Work out the finished part from the listing and answer in its coordinate system (mm). A direction names the side the tool comes from. Round coordinates to 2 decimals unless told otherwise and drop trailing zeros. Write each loop counter-clockwise with the first axis right and the second up, starting at its lowest first coordinate (ties: lowest second). Pieces come first, ordered by that corner, then holes.
1. Find section B-B (x = -13.2). Write down the section's boundary in (y, z).
2. Find section A-A (y = -3). Write down the section's boundary in (x, z), and give its area (3 significant figures).
3. Find section C-C (z = -16). Write down the section's boundary in (x, y), and give its area (3 significant figures).
4. Determine the mould class of faces 1 (the face through (21.58, 3.46, -15.17)), 2 (the face through (-16, 1, -17)), 3 (the face through (-7.6, -7.43, -15.93)) for opening direction X: pulls with the +X half, pulls with the -X half, needs draft (parallel to the pull), parting line crosses it, or undercut.
5. Flat-ended cylindrical pins translate along their axes: pin 1 Ø6 at (x, z) = (-10.5, -16) entering from -Y; pin 2 Ø2.5 at (y, z) = (-3, -16.5) entering from +X; pin 3 Ø6 at (x, y) = (-10.5, -5.5) entering from +Z; pin 4 Ø5 at (y, z) = (-2.5, -16.5) entering from -X. Find the tip coordinate at first contact, or state that the pin passes through.
6. A tool of negligible diameter and unlimited length cuts with its end or side. For faces 4 (the face through (20, 6, -16)), 5 (the face through (-8.2, -3, -16)), 6 (the face through (19.2, -3, -16)), 7 (the face through (6, -6, -16)), from which of +Z, -Z, +X, -X, +Y, -Y can it reach the whole face along a straight path? Write none if from no direction.
7. Find section D-D (y = 3.5). Write down the section's boundary in (x, z).
8. Straight lines are drawn through the part: probe 1 along X at (y, z) = (4.35, -16); probe 2 along Z at (x, y) = (-13.2, 4.1); probe 3 along X at (y, z) = (2.4, -16). For each, find the intervals that lie inside material, in ascending order.
```python
from build123d import *

# Parameters (mm, degrees)
PAD053_DEPTH            = 5
SKETCH104_R             = 2.75
POCKET052_DEPTH         = 8.001
POCKET052_DEPTH_BACK    = 6.001
BODY032_PLACEMENT_ANGLE = 180


with BuildPart() as part:
    # Sketch103 → Pad053 (new body, symmetric)
    with BuildSketch(Plane(origin=(6, -6, 0), x_dir=(1, 0, 0), z_dir=(0, 0, 1))):
        with BuildLine():
            Line((-21.7, 5), (-15.7, 5))
            ThreePointArc((-15.7, 5), (-14.2857864376, 5.5857864376), (-13.7, 7))
            Line((-13.7, 7), (-13.7, 12))
            ThreePointArc((-11.7, 14), (-13.1142135624, 13.4142135624), (-13.7, 12))
            Line((-11.7, 14), (0, 14))
            Line((0, 14), (0, 12))
            Line((0, 12), (-11.7, 12))
            Line((-11.7, 12), (-11.7, 0))
            Line((-11.7, 0), (-23.7, 0))
            Line((-23.7, 0), (-23.7, 3))
            ThreePointArc((-21.7, 5), (-23.1142135624, 4.4142135624), (-23.7, 3))
        make_face()
    extrude(amount=PAD053_DEPTH, both=True)

    # Sketch104 → Pocket052 (cut, two sides)
    with BuildSketch(Plane.XZ) as pocket052_sk:
        with Locations((-12.7, 0)):
            Circle(SKETCH104_R)
    extrude(amount=-POCKET052_DEPTH, mode=Mode.SUBTRACT)
    extrude(pocket052_sk.sketch, amount=POCKET052_DEPTH_BACK, mode=Mode.SUBTRACT)

    # Mirrored024: part across Sketch103 V_Axis


with BuildPart() as part_1:
    add(part.part)
    add(part.part.mirror(Plane(origin=(6, -6, 0), x_dir=(0, 0, 1), z_dir=(1, 0, 0))))


with BuildPart() as part_2:
    # Body032 placement: moved
    add(part_1.part.moved(Location((11.5, 0, -16))).rotate(Axis((11.5, 0, -16), (0, 0, 1)), BODY032_PLACEMENT_ANGLE))


solid = part_2.part
```
Worked answers:
1. outline: (1, -21) - (6, -21) - (6, -18.75) - (1, -18.75) - close; (1, -13.25) - (6, -13.25) - (6, -11) - (1, -11) - close
2. outline: (-8.2, -21) - (-6.2, -21) - (-6.2, -11) - (-8.2, -11) - close; (17.2, -21) - (19.2, -21) - (19.2, -11) - (17.2, -11) - close
2. area: 40.0 mm2
3. outline: (-18.2, 3) arc R2 ccw to (-16.2, 1) - (-15.95, 1) - (-15.95, 6) - (-18.2, 6) - close; (-10.45, 1) - (-10.2, 1) arc R2 cw to (-8.2, -1) - (-8.2, -6) arc R2 ccw to (-6.2, -8) - (17.2, -8) arc R2 ccw to (19.2, -6) - (19.2, -1) arc R2 cw to (21.2, 1) - (21.45, 1) - (21.45, 6) - (17.2, 6) - (17.2, -6) - (-6.2, -6) - (-6.2, 6) - (-10.45, 6) - close; (26.95, 1) - (27.2, 1) arc R2 ccw to (29.2, 3) - (29.2, 6) - (26.95, 6) - close
3. area: 146 mm2
4. face 1: undercut
4. face 2: needs draft
4. face 3: pulls with the -X half
5. pin 1: stops at y = -7.52
5. pin 2: stops at x = 19.2
5. pin 3: stops at z = -11
5. pin 4: stops at x = -8.47
6. face 4: +Z, -Z, +X, -X, +Y
6. face 5: +Z, -Z, -X, -Y
6. face 6: +Z, -Z, +X, -Y
6. face 7: +Z, -Z, +Y
7. outline: (-18.2, -21) - (-6.2, -21) - (-6.2, -11) - (-18.2, -11) - close; (17.2, -21) - (29.2, -21) - (29.2, -11) - (17.2, -11) - close; hole circle Ø5.5 at (-13.2, -16); hole circle Ø5.5 at (24.2, -16)
8. probe 1: x = -18.2 to -15.95, -10.45 to -6.2, 17.2 to 21.45, 26.95 to 29.2
8. probe 2: z = -21 to -18.75, -13.25 to -11
8. probe 3: x = -18.11 to -15.95, -10.45 to -6.2, 17.2 to 21.45, 26.95 to 29.11
